from build123d import *

# Parameters (mm, degrees)
F0_W     = 35.56
F0_H     = 35.56
F0_W_2   = 25.4
F0_H_2   = 25.4
F1_DEPTH = 5.08
F2_W     = 19.812
F2_H     = 4.572
F3_DEPTH = 2.54
F4_W     = 19.812
F4_H     = 4.572
F5_DEPTH = 2.54
F6_W     = 20.32
F6_H     = 5.08
F7_DEPTH = 2.54
F8_W     = 20.32
F8_H     = 5.08
F9_DEPTH = 2.54


with BuildPart() as f1:
    # F0 (on Top) → F1 (new body, symmetric)
    with BuildSketch(Plane.XY):
        Rectangle(F0_W, F0_H)
        Rectangle(F0_W_2, F0_H_2, mode=Mode.SUBTRACT)
    extrude(amount=F1_DEPTH, both=True)

    # F2 (on face) → F3 (join)
    with BuildSketch(Plane(origin=(-17.78, 0, 0), x_dir=(0, -1, 0), z_dir=(-1, 0, 0))):
        Rectangle(F2_W, F2_H)
    extrude(amount=F3_DEPTH)

    # F4 (on face) → F5 (join)
    with BuildSketch(Plane(origin=(0, 17.78, 0), x_dir=(-1, 0, 0), z_dir=(0, 1, 0))):
        Rectangle(F4_W, F4_H)
    extrude(amount=F5_DEPTH)

    # F6 (on face) → F7 (cut)
    with BuildSketch(Plane.YZ.offset(17.78)):
        Rectangle(F6_W, F6_H)
    extrude(amount=-F7_DEPTH, mode=Mode.SUBTRACT)

    # F8 (on face) → F9 (cut)
    with BuildSketch(Plane.XZ.offset(17.78)):
        Rectangle(F8_W, F8_H)
    extrude(amount=-F9_DEPTH, mode=Mode.SUBTRACT)


solid = f1.part
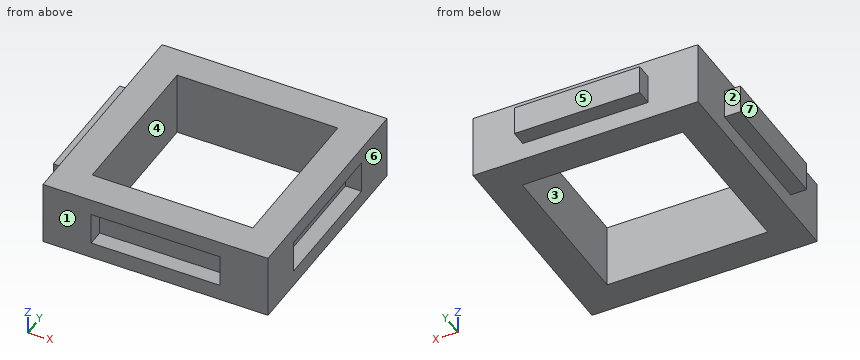
Input: part model. Units: mm. Frame: model coordinates. Face numbers are marked on the shaded views. A direction names the side the tool comes from. Coordinates: 2 decimals unless noted, no trailing zeros. Loops run counter-clockwise (first coordinate to the right, second up) from the corner with the lowest first, then second, coordinate; pieces in that order, holes last. Notation, with made-up numbers: (32, -24.75) -> (59, -24.75) arc R21 cw to (59, -10.75) -> close; hole circle Ø6 at (41.5, -3). An arc over 180 degrees is marked (long way). Write each question's results on one line, items separated by ' | '. Start each with the question number.
Q1. Section B-B, the plane z = -0.75. Return the cut outline in (x, y), plus the area to 3 significant figures.
Q2. Pull-direction query (X, two-part tool) for the marked faces 4, 5, 6 and 7; classes: released by +X, released by -X, zero draft, split by the parting line, or undercut.
Q3. Reachability of the marked faces 1, 2 and 3 from +Z, -Z, +X, -X, +Y, -Y: full face, straight path, thin tool, end or side. Return the list, or none.
Q4. Section C-C, the plane x = -9. Return the cut outline in (y, z).
Q5. Ray query, line 1 (X direction, y = -9, z = 4); line 2 (Y direction, x = -9.5, z = 1.75); line 3 (X direction, y = -2.5, z = 1). Return the intervals inside material, ascending. Write a range as from..to.
Q6. Section A-A, the plane y = -6. Return the cut outline in (x, z), plus the area to 3 significant figures.
Q7. Section D-D, the plane y = -12. Return the cut outline in (x, z).
Q8. Pin query (flat end, axial travel): pin 1 (2 mm diameter, centred on x = -19.5, y = -4.5, fed in from -Z); pin 2 (2.5 mm diameter, centred on y = -3.5, z = -1, fed in from +X); pin 3 (2 mm diameter, centred on x = 3.5, y = 11, fed in from -Z); pin 4 (2 mm diameter, centred on x = -19, y = 0.5, fed in from +Z). Return the tip coordinate at first contact, or that it passes through.
Found:
1) outline: (-20.32, -9.91) -> (-17.78, -9.91) -> (-17.78, -17.78) -> (-10.16, -17.78) -> (-10.16, -15.24) -> (10.16, -15.24) -> (10.16, -17.78) -> (17.78, -17.78) -> (17.78, -10.16) -> (15.24, -10.16) -> (15.24, 10.16) -> (17.78, 10.16) -> (17.78, 17.78) -> (9.91, 17.78) -> (9.91, 20.32) -> (-9.91, 20.32) -> (-9.91, 17.78) -> (-17.78, 17.78) -> (-17.78, 9.91) -> (-20.32, 9.91) -> close; hole (-12.7, -12.7) -> (12.7, -12.7) -> (12.7, 12.7) -> (-12.7, 12.7) -> close | area: 617 mm2
2) face 4: undercut | face 5: zero draft | face 6: released by +X | face 7: released by -X
3) face 1: +Z, -Z, +X, -X, -Y | face 2: +Z, -Z, -X, +Y | face 3: +Z, -Z
4) outline: (-17.78, -5.08) -> (-12.7, -5.08) -> (-12.7, 5.08) -> (-17.78, 5.08) -> (-17.78, 2.54) -> (-15.24, 2.54) -> (-15.24, -2.54) -> (-17.78, -2.54) -> close; (12.7, -5.08) -> (17.78, -5.08) -> (17.78, -2.29) -> (20.32, -2.29) -> (20.32, 2.29) -> (17.78, 2.29) -> (17.78, 5.08) -> (12.7, 5.08) -> close
5) line 1: -17.78..-12.7, 12.7..17.78 | line 2: -15.24..-12.7, 12.7..20.32 | line 3: -20.32..-12.7, 12.7..15.24
6) outline: (-20.32, -2.29) -> (-17.78, -2.29) -> (-17.78, -5.08) -> (-12.7, -5.08) -> (-12.7, 5.08) -> (-17.78, 5.08) -> (-17.78, 2.29) -> (-20.32, 2.29) -> close; (12.7, -5.08) -> (17.78, -5.08) -> (17.78, -2.54) -> (15.24, -2.54) -> (15.24, 2.54) -> (17.78, 2.54) -> (17.78, 5.08) -> (12.7, 5.08) -> close | area: 102 mm2
7) outline: (-17.78, -5.08) -> (-12.7, -5.08) -> (-12.7, 5.08) -> (-17.78, 5.08) -> close; (12.7, -5.08) -> (17.78, -5.08) -> (17.78, 5.08) -> (12.7, 5.08) -> close
8) pin 1: z = -2.29 | pin 2: x = 15.24 | pin 3: through | pin 4: z = 2.29
